Answer from the drawing. Dimensions are ordinates in mm from the lowest x, y and z of the part. Coordinates: 2 decimals unless noted, no trailing zeros. Loops run counter-clockwise (first coordinate to the right, second up) from the corner with the lowest first, then second, coordinate; pieces in that order, holes last. Notation, with made-up numbers: (86, 28) -> (126, 28) arc R18 ccw to (126, 34) -> close; hole circle Ø4 at (50.25, 23.5). An arc over 180 degrees is marked (long way). Answer as CSV lines item,"result".
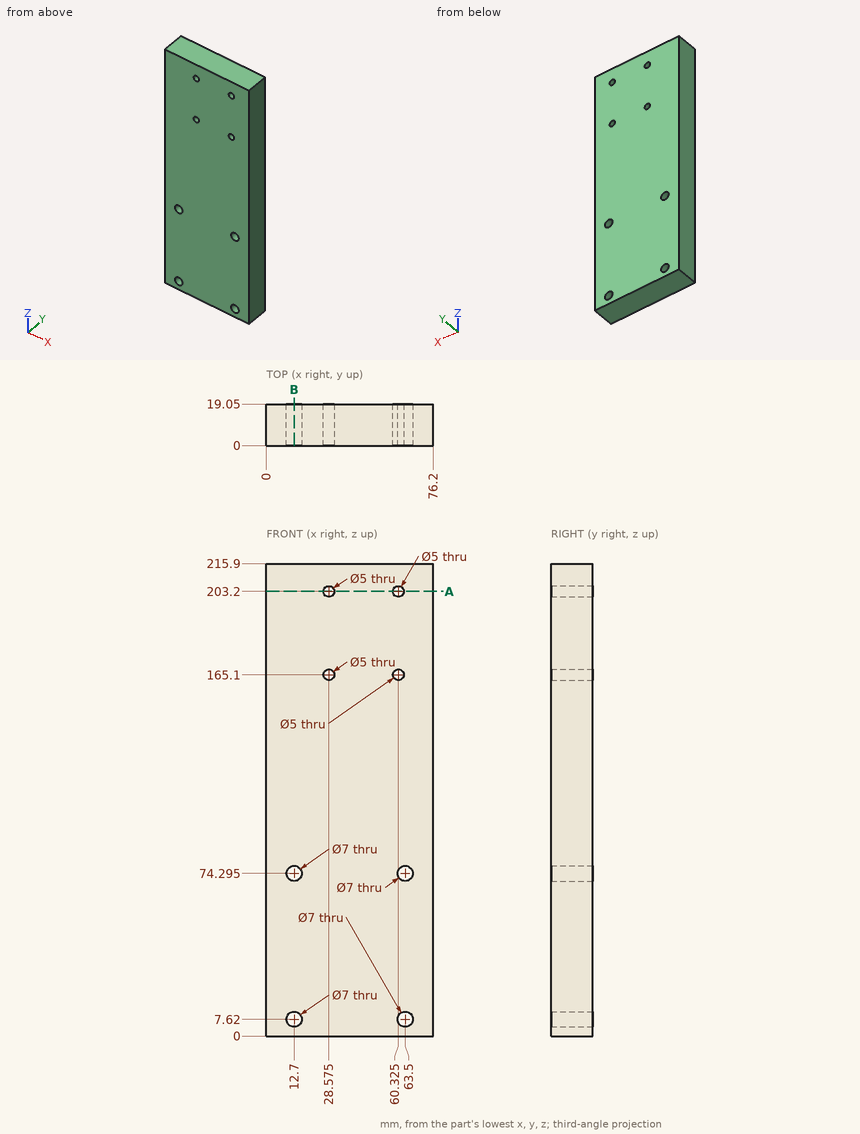
(1) A cutting plane is placed at B-B, the plane x = 12.7. Write down the section's boundary in (y, z) (3 decimals).
Computed values:
outline,"(0, 0) -> (19.05, 0) -> (19.05, 4.12) -> (0, 4.12) -> close; (0, 11.12) -> (19.05, 11.12) -> (19.05, 70.795) -> (0, 70.795) -> close; (0, 77.795) -> (19.05, 77.795) -> (19.05, 215.9) -> (0, 215.9) -> close"
(2) Consider line 1 along X through (y, z) = (14.5, 203.2) (3 decimals); line 2 along Z through (x, y) = (12.7, 6.5) (3 decimals); line 3 along Z through (x, y) = (15, 14.75). Determine where each line is inside the solid, lowest interval first.
Computed values:
line 1,"0 to 26.075, 31.075 to 57.825, 62.825 to 76.2"
line 2,"0 to 4.12, 11.12 to 70.795, 77.795 to 215.9"
line 3,"0 to 4.98, 10.26 to 71.66, 76.93 to 215.9"
(3) A cutting plane is placed at A-A, the plane z = 203.2. Write down the section's boundary in (x, y) (3 decimals), and give its area (3 significant figures).
Computed values:
outline,"(0, 0) -> (26.075, 0) -> (26.075, 19.05) -> (0, 19.05) -> close; (31.075, 0) -> (57.825, 0) -> (57.825, 19.05) -> (31.075, 19.05) -> close; (62.825, 0) -> (76.2, 0) -> (76.2, 19.05) -> (62.825, 19.05) -> close"
area,"1,260 mm2"
(4) Flat-ended cylindrical pins translate along their axes: pin 1 Ø1 at (x, z) = (60.5, 147) entering from -Y; pin 2 Ø5.5 at (x, z) = (12.7, 74.295) entering from +Y. Find the tip coordinate at first contact, or state that the pin passes through.
Computed values:
pin 1,"y = 0"
pin 2,"through"
